Read the model definition and answer for the solid it produces. Units are mm, in the model's axes. A direction names the side the tool comes from. Give positions to 0.01 mm unless a question says otherwise; leave off trailing zeros. Order: outer loops, then holes, each group sorted by start corner. A loop starts at its lowest first (then second) coordinate and runs counter-clockwise, first axis right, second up. Notation, with made-up numbers: (51.5, -1.75) - (73.5, -1.75) arc R19 ccw to (73.5, 22.25) - close; hole circle Ø9 at (77.25, 76). An arc over 180 degrees is marked (long way). One line per item, written item: value. Start each with the question number.
```python
from build123d import *

# Parameters (mm, degrees)
F0_R      = 61.5
F1_DEPTH  = 2
F3_R      = 50.15
F4_R      = 61.5
F6_R      = 36.5
F7_DEPTH  = 5.751
F8_R      = 50.15
F8_R_2    = 36.5
F9_DEPTH  = 2
F10_R     = 2.225
F11_DEPTH = 5.751
F13_DEPTH = 2
F15_DEPTH = 6.55
F17_W     = 6.5
F17_H     = 5.3
F18_DEPTH = 5
F20_W     = 6.5
F20_H     = 5.3
F21_DEPTH = 4
F22_R     = 1


with BuildPart() as f1:
    # F0 (on Top) → F1 (new body)
    with BuildSketch(Plane.XY):
        Circle(F0_R)
    extrude(amount=F1_DEPTH)

    # F3 (on offset) → F5 section 0
    with BuildSketch(Plane.XY.offset(5.75)):
        Circle(F3_R)
    # F4 (on face) → F5 section 1
    with BuildSketch(Plane.XY.offset(2)):
        Circle(F4_R)
    loft()

    # F6 (on face) → F7 (cut, through all)
    with BuildSketch(Plane.XY.offset(5.75)):
        Circle(F6_R)
    extrude(amount=-F7_DEPTH, mode=Mode.SUBTRACT)

    # F8 (on face) → F9 (cut)
    with BuildSketch(Plane.XY.offset(5.75)):
        Circle(F8_R)
        Circle(F8_R_2, mode=Mode.SUBTRACT)
    extrude(amount=-F9_DEPTH, mode=Mode.SUBTRACT)

    # F10 (on face) → F11 (cut, through all)
    with BuildSketch(Plane.XY.offset(5.75)):
        with Locations((0, 42.825)):
            Circle(F10_R)
        with Locations((0, -42.825)):
            Circle(F10_R)
    extrude(amount=-F11_DEPTH, mode=Mode.SUBTRACT)

    # F12 (on face) → F13 (join, through all)
    with BuildSketch(Plane.XY.offset(5.75)):
        with BuildLine():
            Line((-43.1380415063, 6.5), (-46.3969018362, 6.5))
            ThreePointArc((-46.3969018362, 6.5), (-46.85, 0), (-46.3969018362, -6.5))
            Line((-46.3969018362, -6.5), (-43.1380415063, -6.5))
            ThreePointArc((-43.1380415063, -6.5), (-43.625, 0), (-43.1380415063, 6.5))
        make_face()
        with BuildLine():
            Line((43.1380415063, -6.5), (46.3969018362, -6.5))
            ThreePointArc((46.3969018362, -6.5), (46.85, 0), (46.3969018362, 6.5))
            Line((46.3969018362, 6.5), (43.1380415063, 6.5))
            ThreePointArc((43.1380415063, 6.5), (43.625, 0), (43.1380415063, -6.5))
        make_face()
    extrude(amount=-F13_DEPTH)

    # F14 (on face) → F15 (join)
    with BuildSketch(Plane.XY.offset(5.75)):
        with BuildLine():
            Line((-43.1380415063, 6.5), (-46.3969018362, 6.5))
            ThreePointArc((-46.3969018362, 6.5), (-46.85, 0), (-46.3969018362, -6.5))
            Line((-46.3969018362, -6.5), (-43.1380415063, -6.5))
            ThreePointArc((-43.1380415063, -6.5), (-43.625, 0), (-43.1380415063, 6.5))
        make_face()
        with BuildLine():
            Line((43.1380415063, -6.5), (46.3969018362, -6.5))
            ThreePointArc((46.3969018362, -6.5), (46.85, 0), (46.3969018362, 6.5))
            Line((46.3969018362, 6.5), (43.1380415063, 6.5))
            ThreePointArc((43.1380415063, 6.5), (43.625, 0), (43.1380415063, -6.5))
        make_face()
    extrude(amount=F15_DEPTH)

    # F17 (on 3pt) → F18 (cut)
    with BuildSketch(Plane.YZ.offset(-43.1380415063)):
        with Locations((-3.25, 6.4)):
            Rectangle(F17_W, F17_H)
    extrude(amount=-F18_DEPTH, mode=Mode.SUBTRACT)

    # F20 (on 3pt) → F21 (cut)
    with BuildSketch(Plane.YZ.offset(43.1380415063)):
        with Locations((3.25, 6.4)):
            Rectangle(F20_W, F20_H)
    extrude(amount=F21_DEPTH, mode=Mode.SUBTRACT)

    # F22
    f22_edges = [f1.edges().sort_by_distance(p)[0] for p in [
        (44.767472, 6.5, 12.3),
        (-44.767472, -6.5, 12.3),
        (-46.85, 0, 12.3),
        (-43.625, 0, 12.3),
        (43.625, 0, 12.3),
        (46.85, 0, 12.3),
        (43.138042, 6.5, 10.675),
        (-46.396902, -6.5, 10.675),
        (-43.138042, -6.5, 10.675),
        (46.396902, 6.5, 10.675),
        (-44.767472, 6.5, 12.3),
        (44.767472, -6.5, 12.3),
    ]]
    fillet(f22_edges, radius=F22_R)


solid = f1.part
```
1) Find the intervals of material crossed by probe 1 along Y at (x, z) = (0, 1.25); probe 2 along Z at (x, y) = (-47.5, -3.5); probe 3 along X at (y, z) = (4, 9.75), in increasing order. Write a range as from..to.
2) Section A-A on x = 0 is taken. Write down the section's boundary in (y, z).
3) For faces 1 (the flat face through (45, 3, 9.05)), 2 (the cylindrical face through (46.326, -19.208, 4.764)), 3 (the cylindrical face through (-0.29, -40.62, 1.9)), 4 (the flat face through (45, 0, 6)), 5 (the flat face through (26, -26, 0)), determine the directions among +Z, -Z, +X, -X, +Y, -Y from which every point of the face is accessible in a straight line to the end or side of a thin tool.
4) Each of these flat-tipped pins is pushed along its axis until it touches: pin 1 (0.6 mm diameter, centred on x = 45, z = 10.5, fed in from +Y); pin 2 (1 mm diameter, centred on x = 44.5, z = 7, fed in from +Y); pin 3 (4 mm diameter, centred on x = 45.5, y = 4, fed in from -Z); pin 4 (5 mm diameter, centred on x = 24, y = 38, fed in from +Z). Where does it stop, or does it pass through?
5) The mould has two halves that part along Y. Classify faces 6 (the cylindrical face through (28.38, -54.56, 0.99)), 7 (the flat face through (45, -6.5, 8)), 8 (the flat face through (-45, -3, 9.05)): +Y half, -Y half, draft (parallel to the pull), parting line (faces both ways), or undercut.
Solved:
1. probe 1: y = -61.5..-45.05, -40.6..-36.5, 36.5..40.6, 45.05..61.5
1. probe 2: z = 0..3.75
1. probe 3: x = -46.68..-43.44, 43.44..46.68
2. outline: (-61.5, 0) - (-45.05, 0) - (-45.05, 3.75) - (-50.15, 3.75) - (-50.15, 5.75) - (-61.5, 2) - close; (-40.6, 0) - (-36.5, 0) - (-36.5, 3.75) - (-40.6, 3.75) - close; (36.5, 0) - (40.6, 0) - (40.6, 3.75) - (36.5, 3.75) - close; (45.05, 0) - (61.5, 0) - (61.5, 2) - (50.15, 5.75) - (50.15, 3.75) - (45.05, 3.75) - close
3. face 1: +X, +Y
3. face 2: +Z
3. face 3: +Z, -Z
3. face 4: none
3. face 5: -Z, +X, -X, +Y, -Y
4. pin 1: stops at y = 6.5
4. pin 2: stops at y = 0
4. pin 3: stops at z = 0
4. pin 4: stops at z = 3.75
5. face 6: parting line
5. face 7: undercut
5. face 8: draft
